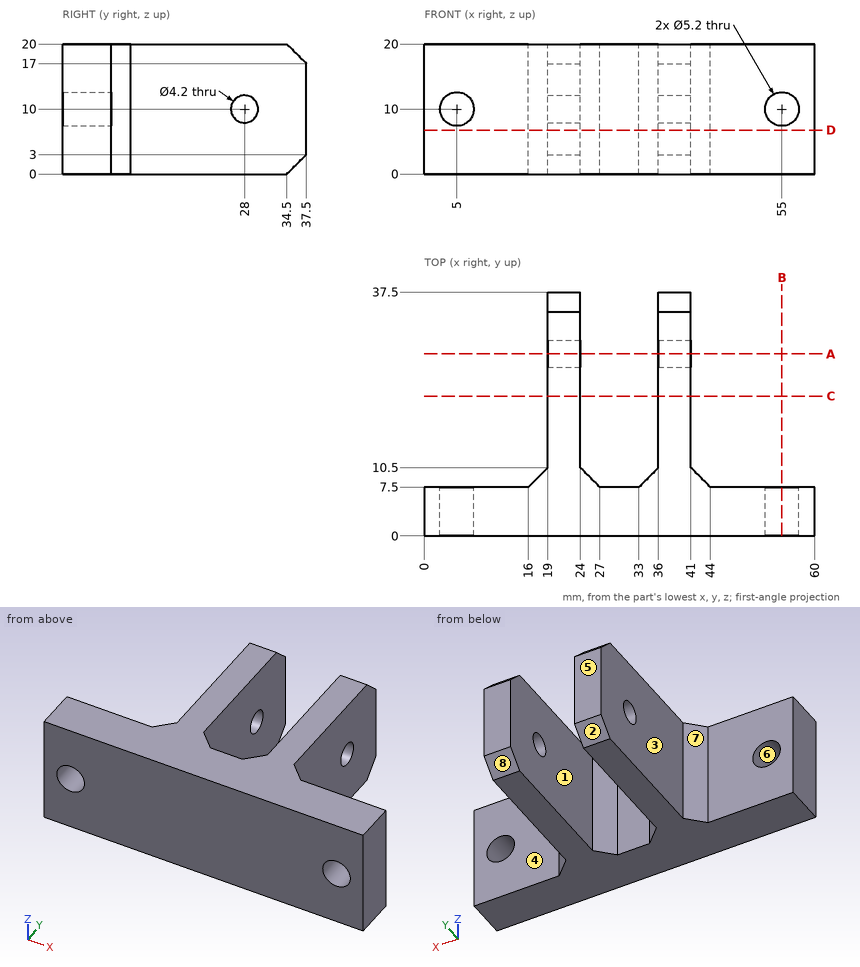
Geometry: see drawing. Coordinates: mm, zero at the bounding-box minimum. A direction names the side the tool comes from. Give positions to 0.01 mm unless a question says otherwise; leave off trailing zeros. Write each loop counter-clockwise with the first axis right and the second up, starting at its lowest first coordinate (ties: lowest second). Pieces come first, ordered by that corner, then holes. Notation, with made-up numbers: (55, -25.75) -> (75, -25.75) arc R28 cw to (75, -0.75) -> close; hole circle Ø4 at (-11, 65). An arc over 180 degrees is marked (long way). Use one line per item in the form item = value. Start each with the question number.
1) Section query D-D on z = 6.75. Return the cut outline in (x, y), then the cut area to 3 significant figures.
2) Set-up query: the marked faces 1, 2, 3, 4 and 5. Return all of +Z, -Z, +X, -X, +Y, -Y with unobstructed straight access to the full face (end or side cutting, diameter ignored); none if empty.
3) Ray query, probe 1 along Z at (x, y) = (20.3, 28); probe 2 along Z at (x, y) = (55, 5); probe 3 along X at (y, z) = (29, 16.5). Return the intervals inside material, ascending. Write a range as from..to.
4) Section query B-B on x = 55. Return the cut outline in (y, z).
5) Section query C-C on y = 21.5. Return the cut outline in (x, z).
6) Section query A-A on y = 28. Return the cut outline in (x, z).
7) Draft query along Z for the marked faces 6, 7 and 8. Return one class per face: pulls with the +Z half, pulls with the -Z half, needs draft (parallel to the pull), parting line crosses it, or undercut.
8) Pin query (flat end, axial travel): pin 1 (12 mm diameter, centred on x = 47.5, z = 16.5, fed in from +Y); pin 2 (3 mm diameter, centred on x = 5, z = 10, fed in from -Y); pin 3 (6 mm diameter, centred on y = 18.5, z = 7, fed in from +X); pin 4 (5 mm diameter, centred on x = 5.5, z = 9.5, fed in from +Y). Return the tip coordinate at first contact, or that it passes through.
Outcome:
q1.outline = (0, 0) -> (60, 0) -> (60, 7.5) -> (44, 7.5) -> (41, 10.5) -> (41, 37.5) -> (36, 37.5) -> (36, 10.5) -> (33, 7.5) -> (27, 7.5) -> (24, 10.5) -> (24, 37.5) -> (19, 37.5) -> (19, 10.5) -> (16, 7.5) -> (0, 7.5) -> close
q1.area = 768 mm^2
q2.face_1 = +Z, -Z, +Y
q2.face_2 = -Z, +X, -X, +Y
q2.face_3 = +Z, -Z, -X, +Y
q2.face_4 = +Z, -Z, +X, +Y
q2.face_5 = +Z, -Z, +X, -X, +Y
q3.probe_1 = 0..7.9, 12.1..20
q3.probe_2 = 0..7.4, 12.6..20
q3.probe_3 = 19..24, 36..41
q4.outline = (0, 0) -> (7.5, 0) -> (7.5, 7.4) -> (0, 7.4) -> close; (0, 12.6) -> (7.5, 12.6) -> (7.5, 20) -> (0, 20) -> close
q5.outline = (19, 0) -> (24, 0) -> (24, 20) -> (19, 20) -> close; (36, 0) -> (41, 0) -> (41, 20) -> (36, 20) -> close
q6.outline = (19, 0) -> (24, 0) -> (24, 7.9) -> (19, 7.9) -> close; (19, 12.1) -> (24, 12.1) -> (24, 20) -> (19, 20) -> close; (36, 0) -> (41, 0) -> (41, 7.9) -> (36, 7.9) -> close; (36, 12.1) -> (41, 12.1) -> (41, 20) -> (36, 20) -> close
q7.face_6 = undercut
q7.face_7 = needs draft
q7.face_8 = pulls with the -Z half
q8.pin_1 = 10
q8.pin_2 = through
q8.pin_3 = 41
q8.pin_4 = 7.5
